```python
from build123d import *

# Parameters (mm, degrees)
F0_W     = 152.4
F0_H     = 114.3
F1_DEPTH = 12.7
F2_W     = 76.2
F2_H     = 114.3
F3_DEPTH = 79.248
F5_DEPTH = 114.301


with BuildPart() as f1:
    # F0 (on Top) → F1 (new body)
    with BuildSketch(Plane.XY):
        with Locations((24.443777, -7.478296)):
            Rectangle(F0_W, F0_H)
    extrude(amount=F1_DEPTH)

    # F2 (on face) → F3 (join)
    with BuildSketch(Plane.XY.offset(12.7)):
        with Locations((24.443777, -7.478296)):
            Rectangle(F2_W, F2_H)
    extrude(amount=F3_DEPTH)

    # F4 (on face) → F5 (cut, through all)
    with BuildSketch(Plane.XZ.offset(64.628296)):
        with BuildLine():
            Line((56.193777, 91.948), (24.443777, 91.948))
            Line((24.443777, 91.948), (24.443777, 60.198))
            ThreePointArc((24.443777, 60.198), (46.894417, 69.49736), (56.193777, 91.948))
        make_face()
        with BuildLine():
            Line((24.443777, 91.948), (-7.306223, 91.948))
            ThreePointArc((-7.306223, 91.948), (1.993136, 69.49736), (24.443777, 60.198))
            Line((24.443777, 60.198), (24.443777, 91.948))
        make_face()
    extrude(amount=-F5_DEPTH, mode=Mode.SUBTRACT)


solid = f1.part
```
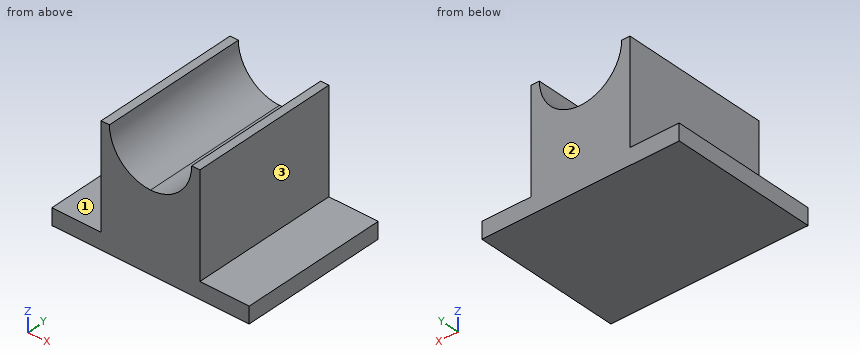
Build history of the part. All positions in model axes, mm. Face numbers are marked on the shaded views. A direction names the side the tool comes from. Give positions to 0.01 mm unless a question says otherwise; leave off trailing zeros. Loops run counter-clockwise (first coordinate to the right, second up) from the corner with the lowest first, then second, coordinate; pieces in that order, holes last.
1) Drop flat-ended pins along their axis: P1, Ø2, axis at x = -20, y = -8, coming from the +Z side; P2, Ø12, axis at x = -23.5, y = -19.5, coming from the -Z side; P3, Ø12, axis at y = -1.5, z = 19.5, coming from the +X side; P4, Ø24, axis at y = -5, z = 39, coming from the -X side. Give the stop position or say it passes through.
Values follow:
P1: stops at z = 12.7
P2: stops at z = 0
P3: stops at x = 62.54
P4: stops at x = -13.66
2) Band-saw the part on C-C on x = 66. List the corners of the cut face in (y, z), then the cut area to 3 significant figures.
Values follow:
outline: (-64.63, 0) - (49.67, 0) - (49.67, 12.7) - (-64.63, 12.7) - close
area: 1,450 mm2
3) 3-axis set-ups, long thin cutter, end or side, ignore diameter. For the marked faces 1, 2 and 3: which of +Z, -Z, +X, -X, +Y, -Y reach the whole face in a straight line?
Values follow:
face 1: +Z, -X, +Y, -Y
face 2: +Z, -Z, +X, -X, +Y
face 3: +Z, +X, +Y, -Y
4) Band-saw the part on D-D on z = 32. List the corners of the cut face in (x, y), then the cut area to 3 significant figures.
Values follow:
outline: (-13.66, -64.63) - (62.54, -64.63) - (62.54, 49.67) - (-13.66, 49.67) - close
area: 8,710 mm2
5) Probe line 1 along X through (y, z) = (-24, 76); line 2 along Z through (x, y) = (-23, -33.5); line 3 along X through (y, z) = (5, 72). List the from-to ranges inside material, lowest first.
Values follow:
line 1: x = -13.66 to -3.01, 51.9 to 62.54
line 2: z = 0 to 12.7
line 3: x = -13.66 to -0.26, 49.14 to 62.54
6) Band-saw the part on B-B on z = 76. List the corners of the cut face in (x, y).
Values follow:
outline: (-13.66, -64.63) - (-3.01, -64.63) - (-3.01, 49.67) - (-13.66, 49.67) - close; (51.9, -64.63) - (62.54, -64.63) - (62.54, 49.67) - (51.9, 49.67) - close
7) Band-saw the part on A-A on y = 12.5. List the corners of the cut face in (x, z), then the cut area to 3 significant figures.
Values follow:
outline: (-51.76, 0) - (100.64, 0) - (100.64, 12.7) - (62.54, 12.7) - (62.54, 91.95) - (56.19, 91.95) arc R31.75 cw to (24.44, 60.2) arc R31.75 cw to (-7.31, 91.95) - (-13.66, 91.95) - (-13.66, 12.7) - (-51.76, 12.7) - close
area: 6,390 mm2
